Autodesk Inventor part; units mm, degrees
ref_plane "YZ Plane" through (0, 0, 0) normal (1, 0, 0) x (0, 1, 0)
ref_plane "XZ Plane" through (0, 0, 0) normal (0, 1, 0) x (-1, 0, 0)
ref_plane "XY Plane" through (0, 0, 0) normal (0, 0, 1) x (1, 0, 0)
sketch "Sketch1" plane through (0, 0, 0) normal (1, 0, 0) x (0, 1, 0)
  circle A0 centre (-9.7574, -19.7073) radius 1.55 construction
  circle A1 centre (0, 0) radius 1.55 construction
  circle A2 centre (-9.7574, -19.7073) radius 2.55
  circle A3 centre (0, 0) radius 2.55
  line L0 (-6.0684, -24.2876) -> (12.7398, 12.1607) construction
  arc A4 (-12.2239, -24.4871) -> (-4.9776, -22.1738) centre (-9.7574, -19.7073) ccw
  circle A5 centre (0, 0) radius 5.7448
  line L1 (-4.9776, -22.1738) -> (5.1052, -2.6344)
  arc A6 (-4.9776, -22.1738) -> (-12.2239, -24.4871) centre (-9.7574, -19.7073) ccw
  line L2 (-14.5372, -17.2408) -> (-5.1904, 2.4623)
  line L3 (0, 0) -> (0, -27.0135) construction
  line L4 (0, 0) -> (-9.7574, -19.7073) construction
  point P0 (-10.1101, -25.5779)
  dimension "d0" = 5.1
  dimension "d1" = 5.1
  dimension "d3" = 11.4897
  dimension "d4" = 5.3787
  dimension "d5" = 21.8076
  dimension "d6" = 21.9875
extrude "Extrusion1" add sketch "Sketch1" along normal blind 4
sketch "Sketch2" plane through (4, 0, 0) normal (1, 0, 0) x (0, 0, -1)
  arc A0 (17.2408, -14.5372) -> (22.1738, -4.9776) centre (19.7073, -9.7574) ccw
  line L0 (22.1738, -4.9776) -> (2.6344, 5.1052)
  arc A1 (2.6344, 5.1052) -> (-2.4623, -5.1904) centre (0, 0) ccw
  line L1 (-2.4623, -5.1904) -> (17.2408, -14.5372) construction
  circle A2 centre (19.7073, -9.7574) radius 2.55 construction
  circle A3 centre (0, 0) radius 2.55 construction
  circle A4 centre (19.7073, -9.7574) radius 2.55 construction
  line L2 (-0.0042, 0.0021) -> (19.7073, -9.7574) construction
  circle A5 centre (13.3596, 13.4709) radius 1
  circle A6 centre (13.3596, 13.4709) radius 4
  line L3 (10.7905, 16.5368) -> (-3.6897, 4.4033)
  arc A7 (2.6344, 5.1052) -> (-2.4623, -5.1904) centre (0, 0) ccw
  line L4 (17.1514, 14.7445) -> (24.806, -8.0448)
  line L5 (-12.5084, -12.3162) -> (6.9664, 27.0174)
  point P0 (-3.6897, 4.4033)
  dimension "d11" = 2
  dimension "d12" = 8
  dimension "d20" = 18
  dimension "d21" = 11.7401
extrude "Extrusion2" add sketch "Sketch2" against normal up to surface (4 mm away)
sketch "Sketch3" plane through (4, 0, 0) normal (1, 0, 0) x (0, 0, -1)
  circle A0 centre (13.3596, 13.4709) radius 1
  circle A1 centre (13.3596, 13.4709) radius 2.5
  point P0 (0, 0)
  dimension "d15" = 5
extrude "Extrusion3" cut sketch "Sketch3" against normal blind 2
properties part number "Kauri modular camera mount nano cam" material "Brass, Soft Yellow"
Work out the finished part from the listing and answer in its coordinate system (mm). A direction names the side the tool comes from. Give positions to 0.01 mm unless a question says otherwise; leave off trailing zeros. Order: outer loops, then holes, each group sorted by start corner. A loop starts at its lowest first (then second) coordinate and runs counter-clockwise, first axis right, second up. Notation, with made-up numbers: (-32.75, 74) -> (26.25, 74) arc R17 ccw to (26.25, 83) -> close; hole circle Ø9 at (86.5, -10). An arc over 180 degrees is marked (long way). Answer as CSV lines item,"result". Start each with the question number.
(1) Each of these flat-tipped pins is pushed along its axis until it touches: pin 1 Ø1 at (x, y) = (1.5, 6.5) entering from -Z; pin 2 Ø3 at (y, z) = (13.47, -13.36) entering from +X; pin 3 Ø1.5 at (x, z) = (3, -8) entering from -Y; pin 4 Ø4 at (y, z) = (0, 0) entering from +X. Where does it stop, or does it pass through?
(2) Consider line 1 along Z through (x, y) = (1.95, 0); line 2 along Z through (x, y) = (2.7, 0.5); line 3 along Y through (x, z) = (1.1, 1). Determine where each line is inside the solid, lowest interval first.
(3) Section B-B, the plane y = -10 is taken. Write down the section's boundary in (x, z).
(4) Section D-D, the plane z = -4 is taken. Write down the section's boundary in (x, y).
(5) For a pull along Y with two mould halves and no side action, classify faces 3 (the cylindrical face through (1.972, -0.809, 5.688)), 4 (the flat face through (4, 1, -9)), 5 (the cylindrical face through (1.97, 1.18, 2.26)) as released by +Y, released by -Y, zero draft, split by the parting line, or undercut.
(6) Which of the six approach directions +Z, -Z, +X, -X, +Y, -Y give full straight-line access (tool end or side, diameter ignored) to faces 1 (the flat face through (2.028, 10.555, -3.652)), 2 (the cylindrical face through (3.014, 15.161, -11.517))?
(7) Section A-A, the plane z = 0 is taken. Write down the section's boundary in (x, y), plus the area to 3 significant figures.
(8) Section C-C, the plane x = 3.35 is taken. Write down the section's boundary in (y, z).
Entries:
1,pin 1,"z = -20.09"
1,pin 2,"x = 2"
1,pin 3,"y = -10.51"
1,pin 4,"through"
2,line 1,"-22.1 to -2.55, 2.55 to 5.74"
2,line 2,"-21.94 to -2.5, 2.5 to 5.72"
2,line 3,"-5.88 to -2.35, 2.35 to 6.66"
3,outline,"(0, -25.08) -> (4, -25.08) -> (4, -22.25) -> (0, -22.25) -> close; (0, -17.17) -> (4, -17.17) -> (4, -7.68) -> (0, -7.68) -> close"
4,outline,"(0, -8.26) -> (4, -8.26) -> (4, 10.85) -> (0, 10.85) -> close"
5,face 3,"split by the parting line"
5,face 4,"zero draft"
5,face 5,"undercut"
6,face 1,"+Z, +X, -X, +Y"
6,face 2,"+X"
7,outline,"(0, -6.36) -> (4, -6.36) -> (4, -2.55) -> (0, -2.55) -> close; (0, 2.55) -> (4, 2.55) -> (4, 7.5) -> (0, 7.5) -> close"
7,area,"35.0 mm²"
8,outline,"(-14.54, -17.24) arc R5.38 ccw to (-8.04, -24.81) -> (14.74, -17.15) arc R4 ccw to (16.54, -10.79) -> (4.4, 3.69) arc R5.74 ccw to (-5.19, 2.46) -> close; hole circle Ø5.1 at (-9.76, -19.71); hole circle Ø5.1 at (0, 0); hole circle Ø5 at (13.47, -13.36)"
